Input: part model. Units: mm. Frame: model coordinates. A direction names the side the tool comes from. Round coordinates to 2 decimals unless told otherwise and drop trailing zeros. Write each loop counter-clockwise with the first axis right and the second up, starting at its lowest first coordinate (ties: lowest second). Pieces come first, ordered by that corner, then holes. Notation, with made-up numbers: M 75,-2.5 L 89,-2.5 A9 cw 89,9.5 Z; hole C 58.25,9.25 d8. An arc over 180 degrees is marked long. Answer as CSV lines item,"result". Start each with the question number.
```python
from build123d import *

# Parameters (mm, degrees)
SKETCH_1_R          = 25
EXTRUDE_1_DEPTH     = 32
SKETCH_2_R          = 27.5
EXTRUDE_2_DEPTH     = 2.5
SKETCH_3_R          = 23
CUT_EXTRUDE_1_DEPTH = 32.5
CHAMFER_1_SIZE      = 3
FILLET_1_R          = 1
FILLET_2_R          = 1
FILLET_3_R          = 1
SKETCH_4_R          = 1.6
CUT_EXTRUDE_2_DEPTH = 32.5
SKETCH_5_R          = 7
CUT_EXTRUDE_3_DEPTH = 10


with BuildPart() as part:
    # Эскиз1 → Бобышка-Вытянуть1 (new body)
    with BuildSketch(Plane.XY):
        Circle(SKETCH_1_R)
    extrude(amount=EXTRUDE_1_DEPTH)

    # Эскиз2 → Бобышка-Вытянуть2 (add)
    with BuildSketch(Plane(origin=(0, 0, 0), x_dir=(-1, 0, 0), z_dir=(0, 0, -1))):
        Circle(SKETCH_2_R)
    extrude(amount=EXTRUDE_2_DEPTH)

    # Эскиз3 → Вырез-Вытянуть1 (cut)
    with BuildSketch(Plane.XY.offset(32)):
        Circle(SKETCH_3_R)
    extrude(amount=-CUT_EXTRUDE_1_DEPTH, mode=Mode.SUBTRACT)

    # Фаска1
    # the kernel refuses this chamfer: 3 mm, written as the material it takes off along each edge
    with BuildSketch(Plane(origin=(0, 0, 32), x_dir=(1, 0, 0), z_dir=(0, -1, 0))) as chamfer_1_piece_1:
        Polygon((25, -CHAMFER_1_SIZE), (25 - CHAMFER_1_SIZE, 0), (25, 0), align=None)
    revolve(axis=Axis((0, 0, 32), (0, 0, 1)), mode=Mode.SUBTRACT)

    # Скругление1
    fillet_1_edges = [part.edges().sort_by_distance(p)[0] for p in [
        (-25, 0, 29),
    ]]
    fillet(fillet_1_edges, radius=FILLET_1_R)

    # Скругление2
    fillet_2_edges = [part.edges().sort_by_distance(p)[0] for p in [
        (-25, 0, 0),
    ]]
    fillet(fillet_2_edges, radius=FILLET_2_R)

    # Скругление3
    fillet_3_edges = [part.edges().sort_by_distance(p)[0] for p in [
        (27.5, 0, -2.5),
    ]]
    fillet(fillet_3_edges, radius=FILLET_3_R)

    # Эскиз4 → Вырез-Вытянуть2 (cut)
    with BuildSketch(Plane(origin=(0, 0, -2.5), x_dir=(-1, 0, 0), z_dir=(0, 0, -1))):
        Circle(SKETCH_4_R)
    extrude(amount=-CUT_EXTRUDE_2_DEPTH, mode=Mode.SUBTRACT)

    # Эскиз5 → Вырез-Вытянуть3 (cut)
    with BuildSketch(Plane(origin=(0, 0, -2.5), x_dir=(-1, 0, 0), z_dir=(0, 0, -1))):
        Circle(SKETCH_5_R)
    extrude(amount=-CUT_EXTRUDE_3_DEPTH, mode=Mode.SUBTRACT)


solid = part.part
```
Item 1: Access query for faces 1 (the face through (-10.1, -24.3, 0)), 2 (the face through (5.961, -26.846, -0.74)). Directions: +Z, -Z, +X, -X, +Y, -Y. A direction counts if a zero-diameter tool reaches every point of the face in a straight line with its end or side. Return the directions, or none.
Item 2: Line query: line 1 (Y direction, x = 0, z = 9); line 2 (Y direction, x = 0, z = -1.3); line 3 (Z direction, x = -8.5, y = -13). Output: solid intervals per line, ascending. Write a range as [from, to].
Item 3: Pin query (flat end, axial travel): pin 1 Ø6 at (y, z) = (0.5, 6) entering from +X; pin 2 Ø10 at (y, z) = (9, 2) entering from +X; pin 3 Ø16.5 at (x, y) = (-3.5, -6) entering from +Z. Return the tip coordinate at first contact, or that it passes through.
Item 4: Cut plane A-A, the plane z = 9. Return loops of the section in (x, y), plus the area to 3 significant figures.
Item 5: Draft query along X for faces 3 (the face through (23.846, 7.509, 14.6)), 4 (the face through (-6, -6, -2.5)), 5 (the face through (4.8, 5.4, -0.5)), 6 (the face through (-6.466, -2.681, -1.514)). Return one class per face: +X half, -X half, draft (parallel to the pull), parting line (faces both ways), or undercut.
Results list:
1,face 1,"+Z"
1,face 2,"+Z, -Z"
2,line 1,"[-25, -23], [23, 25]"
2,line 2,"[-27.5, -7], [7, 27.5]"
2,line 3,"[-2.5, -0.5]"
3,pin 1,"x = 25"
3,pin 2,"x = 27.14"
3,pin 3,"z = -0.5"
4,outline,"C 0,0 d50; hole C 0,0 d46"
4,area,"302 mm²"
5,face 3,"parting line"
5,face 4,"draft"
5,face 5,"undercut"
5,face 6,"undercut"
